```python
from build123d import *

# Parameters (mm, degrees)
EXTRUDE_THIN1_DEPTH = 88.9
SKETCH2_R           = 4.22275
CUT_EXTRUDE2_DEPTH  = 5.08
SKETCH3_W           = 18.017998
SKETCH3_H           = 38.7985
BOSS_EXTRUDE1_DEPTH = 5.08
SKETCH4_W           = 18.017998
SKETCH4_H           = 38.7985
BOSS_EXTRUDE2_DEPTH = 5.08


with BuildPart() as part:
    # Sketch1 → Extrude-Thin1 (new body)
    with BuildSketch(Plane.XY):
        Polygon((-6.468999, 26.06675), (6.468999, 26.06675), (6.468999, -26.06675), (-6.468999, -26.06675), (-6.468999, -31.14675), (11.548999, -31.14675), (11.548999, 31.14675), (-6.468999, 31.14675), align=None)
    extrude(amount=EXTRUDE_THIN1_DEPTH)

    # Sketch2 → Cut-Extrude2 (cut)
    with BuildSketch(Plane.ZY.offset(-6.468999)):
        with Locations((44.45, 0)):
            Circle(SKETCH2_R)
    extrude(amount=-CUT_EXTRUDE2_DEPTH, mode=Mode.SUBTRACT)

    # Sketch3 → Boss-Extrude1 (add)
    with BuildSketch(Plane.XY.offset(88.9)):
        with Locations((2.54, 11.7475)):
            Rectangle(SKETCH3_W, SKETCH3_H)
    extrude(amount=-BOSS_EXTRUDE1_DEPTH)

    # Sketch4 → Boss-Extrude2 (add)
    with BuildSketch(Plane(origin=(0, 0, 0), x_dir=(-1, 0, 0), z_dir=(0, 0, -1))):
        with Locations((-2.54, -11.7475)):
            Rectangle(SKETCH4_W, SKETCH4_H)
    extrude(amount=-BOSS_EXTRUDE2_DEPTH)


solid = part.part
```
Can you work these out from the model? Positions are in its coordinate system, mm. A direction names the side the tool comes from. Round coordinates to 2 decimals unless told otherwise and drop trailing zeros. Loops run counter-clockwise (first coordinate to the right, second up) from the corner with the lowest first, then second, coordinate; pieces in that order, holes last. Notation, with made-up numbers: M -7,34 L 22,34 A18 ccw 22,66 Z; hole C 30,72.25 d3. An arc over 180 degrees is marked long. Write item = value, one per line. Start each with the question number.
(1) I'm going to push flat-ended pins straight in: P1, Ø3, axis at x = -1.5, y = -11, coming from the -Z side; P2, Ø6.5, axis at x = 2, y = 11.5, coming from the -Z side; P3, Ø15.5, axis at y = -7.5, z = 35, coming from the -X side. Where does each tip first touch, or does it pass through?
(2) Suppose I cut it at C-C on z = 28. Write out the boundary of the cut face in (x, y).
(3) Which directions (+Z, -Z, +X, -X, +Y, -Y) give clear straight access to the entire face, cutting with the end or side of a thin tool? Please do faces 1 (the face through (0, 26.067, 41)), 2 (the face through (0, -7.652, 86)), 3 (the face through (0, -9, 5.08)).
(4) Suppose I cut it at D-D on y = -20. Write out the boundary of the cut face in (x, z), plus the area to 3 significant figures.
(5) Suppose I cut it at B-B on x = -2.75. Write out the boundary of the cut face in (y, z).
(6) Suppose I cut it at A-A on y = 0. Write out the boundary of the cut face in (x, z).
(7) If we mould it in two halves opening along Y, with no side actions, what happens to faces 4 (the face through (0, 7.652, 3)), 5 (the face through (2, 7, 88.9)), 6 (the face through (3, 31.147, 44))? For each: released by +Y, released by -Y, zero draft, split by the parting line, or undercut.
(8) I need wall thicknesses on line 1 along Z through (x, y) = (-5.25, 0.5); line 2 along Y through (x, z) = (-0.75, 10.5); line 3 along Y through (x, z) = (4.25, 85.5). Which ranges of each line are inside material? Lowest first, please.
Answer block:
q1.P1 = 0
q1.P2 = 83.82
q1.P3 = 6.47
q2.outline = M -6.47,-31.15 L 11.55,-31.15 L 11.55,31.15 L -6.47,31.15 L -6.47,26.07 L 6.47,26.07 L 6.47,-26.07 L -6.47,-26.07 Z
q3.face_1 = -Z, -X
q3.face_2 = +Z, -X
q3.face_3 = -X
q4.outline = M -6.47,0 L 11.55,0 L 11.55,88.9 L 6.47,88.9 L 6.47,5.08 L -6.47,5.08 Z
q4.area = 517 mm²
q5.outline = M -31.15,0 L 7.65,0 L 7.65,5.08 L -26.07,5.08 L -26.07,88.9 L -31.15,88.9 Z; M -7.65,83.82 L 26.07,83.82 L 26.07,0 L 31.15,0 L 31.15,88.9 L -7.65,88.9 Z
q6.outline = M -6.47,0 L 11.55,0 L 11.55,40.23 L 6.47,40.23 L 6.47,5.08 L -6.47,5.08 Z; M -6.47,83.82 L 6.47,83.82 L 6.47,48.67 L 11.55,48.67 L 11.55,88.9 L -6.47,88.9 Z
q7.face_4 = undercut
q7.face_5 = zero draft
q7.face_6 = released by +Y
q8.line_1 = 0 to 5.08, 83.82 to 88.9
q8.line_2 = -31.15 to -26.07, 26.07 to 31.15
q8.line_3 = -31.15 to -26.07, -7.65 to 31.15
